from build123d import *

# Parameters (mm, degrees)
SKETCH2_W           = 108
SKETCH2_H           = 70
BOSS_EXTRUDE1_DEPTH = 3
SKETCH7_W           = 108
SKETCH7_H           = 70
SKETCH7_W_2         = 102
SKETCH7_H_2         = 64
BOSS_EXTRUDE4_DEPTH = 25
SKETCH16_W          = 2
SKETCH16_H          = 10
SKETCH16_W_2        = 8
SKETCH16_H_2        = 3
SKETCH16_W_3        = 4
SKETCH16_H_3        = 2
BOSS_EXTRUDE5_DEPTH = 22.8
SKETCH19_W          = 6
SKETCH19_H          = 19.4
CUT_EXTRUDE10_DEPTH = 1
SKETCH18_R          = 1.5
SKETCH18_W          = 15.3
SKETCH18_H          = 35.4
CUT_EXTRUDE9_DEPTH  = 79.242054464
BOSS_EXTRUDE6_START = 1.5
SKETCH20_W          = 6
SKETCH20_H          = 10
SKETCH20_R          = 1.5
SKETCH20_R_2        = 2
BOSS_EXTRUDE6_DEPTH = 1.5
SKETCH21_W          = 9
SKETCH21_H          = 6
CUT_EXTRUDE11_DEPTH = 1
SKETCH23_W          = 2.627
SKETCH23_H          = 3.127
SKETCH23_W_2        = 12.754
SKETCH23_H_2        = 6
CUT_EXTRUDE13_DEPTH = 2
SKETCH24_R          = 6.15
SKETCH24_R_2        = 3
CUT_EXTRUDE14_DEPTH = 80.251618827
SKETCH28_W          = 21
SKETCH28_H          = 3
CUT_EXTRUDE15_DEPTH = 5
SKETCH31_W          = 12
SKETCH31_H          = 18
SKETCH31_R          = 3.25
BOSS_EXTRUDE8_DEPTH = 28
FILLET1_R           = 2
CUT_EXTRUDE17_DEPTH = 10


with BuildPart() as part:
    # Sketch2 → Boss-Extrude1 (new body)
    with BuildSketch(Plane(origin=(0, 0, 0), x_dir=(1, 0, 0), z_dir=(0, 1, 0))):
        with Locations((-7.038444533, 7.084764176)):
            Rectangle(SKETCH2_W, SKETCH2_H)
    extrude(amount=BOSS_EXTRUDE1_DEPTH)

    # Sketch7 → Boss-Extrude4 (add)
    with BuildSketch(Plane(origin=(0, 0, 0), x_dir=(-1, 0, 0), z_dir=(0, -1, 0))):
        with Locations((7.038444533, 7.084764176)):
            Rectangle(SKETCH7_W, SKETCH7_H)
        with Locations((7.038444533, 7.084764176)):
            Rectangle(SKETCH7_W_2, SKETCH7_H_2, mode=Mode.SUBTRACT)
    extrude(amount=BOSS_EXTRUDE4_DEPTH)

    # Sketch16 → Boss-Extrude5 (add)
    with BuildSketch(Plane.XZ):
        with Locations((-16.038444533, 3.415235824)):
            Rectangle(SKETCH16_W, SKETCH16_H)
        Polygon((-58.038444533, 14.915235824), (-55.038444533, 14.915235824), (-55.038444533, 21.915235824), (-55.038444533, 24.915235824), (-58.038444533, 24.915235824), align=None)
        with Locations((-51.038444533, 23.415235824)):
            Rectangle(SKETCH16_W_2, SKETCH16_H_2)
        with Locations((-17.038444533, -2.584764176)):
            Rectangle(SKETCH16_W_3, SKETCH16_H_3)
    extrude(amount=BOSS_EXTRUDE5_DEPTH)

    # Sketch19 → Cut-Extrude10 (cut)
    with BuildSketch(Plane.XZ):
        with Locations((-52.538444533, -7.084764176)):
            Rectangle(SKETCH19_W, SKETCH19_H)
    extrude(amount=-CUT_EXTRUDE10_DEPTH, mode=Mode.SUBTRACT)

    # Sketch18 → Cut-Extrude9 (cut, through all)
    with BuildSketch(Plane.XZ):
        with Locations(Location((-52.038444533, -22.284764176, 0), (0, 0, 270))):
            Circle(SKETCH18_R)
        with Locations(Location((-23.538444533, -22.284764176, 0), (0, 0, 270))):
            Circle(SKETCH18_R)
        with Locations(Location((-23.538444533, 8.115235824, 0), (0, 0, 270))):
            Circle(SKETCH18_R)
        with Locations(Location((-52.038444533, 8.115235824, 0), (0, 0, 270))):
            Circle(SKETCH18_R)
        with Locations((-39.688444533, -7.084764176)):
            Rectangle(SKETCH18_W, SKETCH18_H)
    extrude(amount=-CUT_EXTRUDE9_DEPTH, mode=Mode.SUBTRACT)

    # Sketch20 → Boss-Extrude6 (add)
    # profile 1 of 4: a face of its own
    with BuildSketch(Plane.XZ.offset(BOSS_EXTRUDE6_START)):
        with Locations((-52.538444533, 7.615235824)):
            Rectangle(SKETCH20_W, SKETCH20_H)
        with Locations(Location((-52.038444533, 8.115235824, 0), (0, 0, 270))):
            Circle(SKETCH20_R, mode=Mode.SUBTRACT)
    # profile 2 of 4: a face of its own
    with BuildSketch(Plane.XZ.offset(BOSS_EXTRUDE6_START)):
        with Locations((-52.538444533, -21.784764176)):
            Rectangle(SKETCH20_W, SKETCH20_H)
        with Locations(Location((-52.038444533, -22.284764176, 0), (0, 0, 270))):
            Circle(SKETCH20_R_2, mode=Mode.SUBTRACT)
    # profile 3 of 4: a face of its own
    with BuildSketch(Plane.XZ.offset(BOSS_EXTRUDE6_START)):
        with Locations((-23.038444533, -21.784764176)):
            Rectangle(SKETCH20_W, SKETCH20_H)
        with Locations(Location((-23.538444533, -22.284764176, 0), (0, 0, 270))):
            Circle(SKETCH20_R_2, mode=Mode.SUBTRACT)
    # profile 4 of 4: a face of its own
    with BuildSketch(Plane.XZ.offset(BOSS_EXTRUDE6_START)):
        with Locations((-23.038444533, 7.615235824)):
            Rectangle(SKETCH20_W, SKETCH20_H)
        with Locations(Location((-23.538444533, 8.115235824, 0), (0, 0, 270))):
            Circle(SKETCH20_R_2, mode=Mode.SUBTRACT)
    extrude(amount=-BOSS_EXTRUDE6_DEPTH)

    # Sketch21 → Cut-Extrude11 (cut)
    with BuildSketch(Plane.XZ.offset(-3)):
        with Locations((-0.538444533, 7.615235824)):
            Rectangle(SKETCH21_W, SKETCH21_H)
    extrude(amount=CUT_EXTRUDE11_DEPTH, mode=Mode.SUBTRACT)

    # Sketch23 → Cut-Extrude13 (cut)
    with BuildSketch(Plane.XZ):
        with Locations((-0.538444533, 3.051735824)):
            Rectangle(SKETCH23_W, SKETCH23_H)
        with Locations((-0.538444533, 7.615235824)):
            Rectangle(SKETCH23_W_2, SKETCH23_H_2)
    extrude(amount=-CUT_EXTRUDE13_DEPTH, mode=Mode.SUBTRACT)

    # Sketch24 → Cut-Extrude14 (cut, through all)
    with BuildSketch(Plane(origin=(0, 3, 0), x_dir=(1, 0, 0), z_dir=(0, 1, 0))):
        with Locations(Location((1.111555467, 18.634764176, 0), (0, 0, 270))):
            Circle(SKETCH24_R)
        with Locations(Location((23.961555467, -7.615235824, 0), (0, 0, 270))):
            Circle(SKETCH24_R_2)
    extrude(amount=-CUT_EXTRUDE14_DEPTH, mode=Mode.SUBTRACT)

    # Sketch28 → Cut-Extrude15 (cut)
    with BuildSketch(Plane.XZ.offset(25)):
        with Locations((24.461555467, 26.415235824)):
            Rectangle(SKETCH28_W, SKETCH28_H)
    extrude(amount=-CUT_EXTRUDE15_DEPTH, mode=Mode.SUBTRACT)

    # Sketch31 → Boss-Extrude8 (add)
    # profile 1 of 2: a face of its own
    with BuildSketch(Plane.XZ.offset(25)):
        with Locations((-67.038444533, -7.084764176)):
            Rectangle(SKETCH31_W, SKETCH31_H)
        with Locations(Location((-65.538444533, -7.084764176, 0), (0, 0, 270))):
            Circle(SKETCH31_R, mode=Mode.SUBTRACT)
    # profile 2 of 2: a face of its own
    with BuildSketch(Plane.XZ.offset(25)):
        with Locations((52.961555467, -7.084764176)):
            Rectangle(SKETCH31_W, SKETCH31_H)
        with Locations(Location((51.461555467, -7.084764176, 0), (0, 0, 90))):
            Circle(SKETCH31_R, mode=Mode.SUBTRACT)
    extrude(amount=-BOSS_EXTRUDE8_DEPTH)

    # Fillet1
    fillet1_edges = [part.edges().sort_by_distance(p)[0] for p in [
        (-73.038444533, -11, -16.084764176),
        (-73.038444533, -11, 1.915235824),
        (58.961555467, -11, 1.915235824),
        (58.961555467, -11, -16.084764176),
    ]]
    fillet(fillet1_edges, radius=FILLET1_R)

    # Sketch32 → Cut-Extrude17 (cut)
    with BuildSketch(Plane(origin=(0, 3, 0), x_dir=(1, 0, 0), z_dir=(0, 1, 0))):
        Polygon((-60.288444533, 4.053675263), (-60.288444533, 10.115853089), (-65.538444533, 13.146942003), (-70.788444533, 10.115853089), (-70.788444533, 4.053675263), (-65.538444533, 1.02258635), align=None)
        Polygon((51.461555467, 1.02258635), (46.211555467, 4.053675263), (46.211555467, 10.115853089), (51.461555467, 13.146942003), (56.711555467, 10.115853089), (56.711555467, 4.053675263), align=None)
    extrude(amount=-CUT_EXTRUDE17_DEPTH, mode=Mode.SUBTRACT)


solid = part.part
Design review of the part built by this model. Coordinates are the model's own, in mm. A direction names the side the tool comes from. Give positions to 0.01 mm unless a question says otherwise; leave off trailing zeros. Loops run counter-clockwise (first coordinate to the right, second up) from the corner with the lowest first, then second, coordinate; pieces in that order, holes last. Notation, with made-up numbers: M 48.25,18.25 L 62.25,18.25 A20 cw 62.25,33.25 Z; hole C 89.25,-24 d7. An arc over 180 degrees is marked long. One line per question, with ' | ' between items. Start each with the question number.
1. To check wall thickness, follow L1, parallel to X at y = -11.75, z = -0.5; L2, parallel to X at y = -16.25, z = 5; L3, parallel to X at y = -7.75, z = 18.5. State the ranges of each line that lie inside material, in increasing order.
2. Add section D-D (z = -28.5). Write out the cut boundary in (x, y).
3. Add section A-A (y = -14.75). Give the number of separate pieces and of enclosed holes in the cut face, plus the area to 3 significant figures.
4. For faces 1 (the face through (46.212, -2, -7)), 2 (the face through (-40, 1, 10.615)), 3 (the face through (43.962, -12, -7)), list the 3-axis set-ups (+Z, -Z, +X, -X, +Y, -Y) from which the entire face can be reached by the end or side of a thin tool; tool diameter is ignored.
5. Add section C-C (x = -38). Write out the cut boundary in (y, z).
6. Insertion check: P1, Ø8, axis at x = -14, z = -32.5, coming from the -Y side; P2, Ø4, axis at x = -23.54, z = -22.28, coming from the +Y side; P3, Ø1.5, axis at y = -15.5, z = 6.5, coming from the +X side; P4, Ø1.8, axis at x = -22, z = -21.5, coming from the -Y side. Each pin has a flat end and moves straight along its axis. Give the tip position at first contact, or say it passes through.
7. Add section B-B (x = 33.5). Write out the cut boundary in (y, z).
8. The part is to be moulded in two halves that separate along Z. For faces 4 (the face through (-22.5, 1.5, 9.2)), 5 (the face through (-6, -11, 27.915)), 6 (the face through (13.962, -23, 26)), say which applies: released by +Z, released by -Z, zero draft, split by the parting line, or undercut.
Worked out:
1) L1: x = -73.04 to -58.04, -17.04 to -15.04, 43.96 to 58.96 | L2: x = -61.04 to -58.04, -17.04 to -15.04, 43.96 to 46.96 | L3: x = -61.04 to -55.04, 43.96 to 46.96
2) outline: M -61.04,-25 L -58.04,-25 L -58.04,0 L 43.96,0 L 43.96,-25 L 46.96,-25 L 46.96,3 L -61.04,3 Z
3) separate pieces: 2 | enclosed holes: 3 | area: 1,480 mm²
4) face 1: +Y | face 2: +Y, -Y | face 3: -Y
5) outline: M -25,-42.08 L 3,-42.08 L 3,-24.78 L 0,-24.78 L 0,-39.08 L -25,-39.08 Z; M -25,24.92 L 0,24.92 L 0,10.62 L 3,10.62 L 3,27.92 L -25,27.92 Z
6) P1: stops at y = 0 | P2: stops at y = 3 | P3: stops at x = 46.96 | P4: stops at y = -1.5
7) outline: M -25,-42.08 L 3,-42.08 L 3,27.92 L -20,27.92 L -20,24.92 L 0,24.92 L 0,-39.08 L -25,-39.08 Z
8) face 4: undercut | face 5: released by +Z | face 6: zero draft
